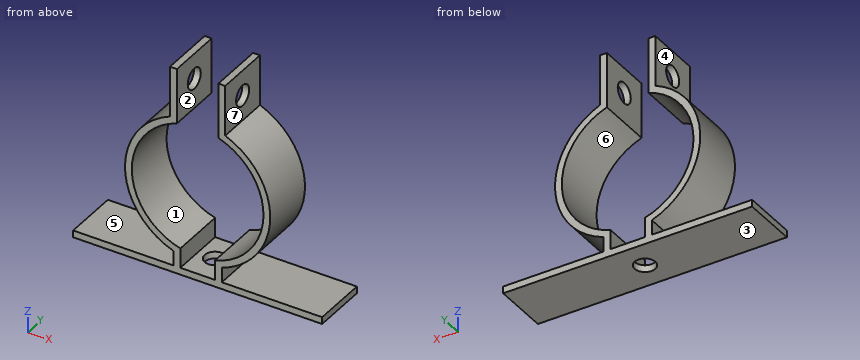
```python
from build123d import *

# Parameters (mm, degrees)
BOSS_EXTRUDE1_DEPTH = 25.4
SKETCH2_R           = 4.7625
CUT_EXTRUDE1_DEPTH  = 25.4
SKETCH3_R           = 4.7625
CUT_EXTRUDE2_DEPTH  = 25.4


with BuildPart() as part:
    # Sketch1 → Boss-Extrude1 (new body)
    with BuildSketch(Plane(origin=(0, 0, 0), x_dir=(1, 0, 0), z_dir=(0, 1, 0))):
        with BuildLine():
            Line((0, 0), (0, 3.175))
            Line((0, 3.175), (114.3, 3.175))
            Line((114.3, 3.175), (114.3, 0))
            Line((114.3, 0), (68.2625, 0))
            Line((68.2625, 0), (68.2625, -6.774088247))
            ThreePointArc((68.2625, -6.774088247), (90.477013576, -37.368879188), (69.8246, -69.03911221))
            Line((69.8246, -69.03911221), (69.8246, -92.290964713))
            Line((69.8246, -92.290964713), (66.675, -92.290964713))
            Line((66.675, -92.290964713), (66.675, -66.890964713))
            ThreePointArc((66.675, -66.890964713), (87.364626112, -37.37586168), (65.0875, -9.03981418))
            Line((65.0875, -9.03981418), (65.0875, 0))
            Line((65.0875, 0), (49.2125, 0))
            Line((49.2125, 0), (49.2125, -9.03981418))
            ThreePointArc((49.2125, -9.03981418), (26.935373888, -37.37586168), (47.625, -66.890964713))
            Line((47.625, -66.890964713), (47.625, -92.290964713))
            Line((47.625, -92.290964713), (44.45, -92.290964713))
            Line((44.45, -92.290964713), (44.45, -69.028659115))
            ThreePointArc((44.45, -69.028659115), (23.823333687, -37.35515016), (46.0375, -6.774088247))
            Line((46.0375, -6.774088247), (46.0375, 0))
            Line((46.0375, 0), (0, 0))
        make_face()
    extrude(amount=BOSS_EXTRUDE1_DEPTH)

    # Sketch2 → Cut-Extrude1 (cut)
    with BuildSketch(Plane(origin=(69.8246, 0, 0), x_dir=(0, 0, -1), z_dir=(1, 0, 0))):
        with Locations((-80.665038461, 12.7)):
            Circle(SKETCH2_R)
    extrude(amount=-CUT_EXTRUDE1_DEPTH, mode=Mode.SUBTRACT)

    # Sketch3 → Cut-Extrude2 (cut)
    with BuildSketch(Plane(origin=(0, 0, -3.175), x_dir=(-1, 0, 0), z_dir=(0, 0, -1))):
        with Locations((-57.15, 12.7)):
            Circle(SKETCH3_R)
    extrude(amount=-CUT_EXTRUDE2_DEPTH, mode=Mode.SUBTRACT)


solid = part.part
```
Can you work these out from the model? Positions are in its coordinate system, mm. Face numbers are marked on the shaded views. A direction names the side the tool comes from. Coordinates: 2 decimals unless noted, no trailing zeros. Order: outer loops, then holes, each group sorted by start corner. A loop starts at its lowest first (then second) coordinate and runs counter-clockwise, first axis right, second up.
1. I need wall thicknesses on line 1 (Z direction, x = 75.5, y = 16) (3 decimals); line 2 (Z direction, x = 47, y = 15.75) (3 decimals); line 3 (X direction, y = 13, z = 2). Which ranges of each line are inside material? Lowest first, please.
2. If we section it at B-B (x = 57.15): Please give me the cut outline in (y, z) (1 decimal).
3. If we section it at C-C (z = 56.5): Please give me the cut outline in (x, y), then the cut area to 3 significant figures.
4. For the marked faces 4, 5, 6 and 7, which set-ups out of +Z, -Z, +X, -X, +Y, -Y let a thin tool reach every point of the face, with its end or its side?
5. If we section it at A-A (y = 12.7): Give the number of separate pieces and of enclosed holes in the cut face, then the cut area to 3 significant figures.
6. Thinking about a two-plate mould opening in Z: for the marked faces 1, 2 and 3, which applies, +Z half, -Z half, draft (parallel to the pull), parting line (faces both ways), or undercut?
7. I'm going to push flat-ended pins straight in: pin 1 (7.5 mm diameter, centred on y = 12.7, z = 80.67, fed in from -X); pin 2 (6 mm diameter, centred on y = 15.5, z = 12.5, fed in from -X); pin 3 (2 mm diameter, centred on y = 11.5, z = 5, fed in from +X); pin 4 (7.5 mm diameter, centred on x = 29.5, y = 16, fed in from +Z). Where does each tip first touch, or does it pass through?
8. If we section it at D-D (x = 40): Please give me the cut outline in (y, z) (3 decimals).
Entries:
1. line 1: z = -3.175 to 0, 10.372 to 14.186, 62.223 to 66.038
1. line 2: z = -3.175 to 9.734, 66.676 to 77.007, 84.323 to 92.291
1. line 3: x = 46.04 to 49.21, 65.09 to 68.26
2. outline: (0, -3.2) - (7.9, -3.2) - (7.9, 0) - (0, 0) - close; (17.5, -3.2) - (25.4, -3.2) - (25.4, 0) - (17.5, 0) - close
3. outline: (29.28, 0) - (33.09, 0) - (33.09, 25.4) - (29.28, 25.4) - close; (81.21, 0) - (85.02, 0) - (85.02, 25.4) - (81.21, 25.4) - close
3. area: 193 mm2
4. face 4: +Z, -X, +Y, -Y
4. face 5: -X, +Y, -Y
4. face 6: +Y, -Y
4. face 7: +Z, +X, +Y, -Y
5. separate pieces: 4
5. enclosed holes: 0
5. area: 967 mm2
6. face 1: undercut
6. face 2: draft
6. face 3: -Z half
7. pin 1: passes through
7. pin 2: stops at x = 32.74
7. pin 3: stops at x = 68.26
7. pin 4: stops at z = 61.45
8. outline: (0, -3.175) - (25.4, -3.175) - (25.4, 0) - (0, 0) - close; (0, 9.617) - (25.4, 9.617) - (25.4, 13.315) - (0, 13.315) - close; (0, 63.095) - (25.4, 63.095) - (25.4, 66.793) - (0, 66.793) - close
